Design review of the part built by this model. Coordinates are the model's own, in mm. A direction names the side the tool comes from. Coordinates: 2 decimals unless noted, no trailing zeros. Order: outer loops, then holes, each group sorted by start corner. A loop starts at its lowest first (then second) coordinate and runs counter-clockwise, first axis right, second up. Notation, with made-up numbers: (68, -26.75) - (108, -26.75) arc R8 ccw to (108, -13.75) - close; hole circle Ø2 at (-37, -38.5). An arc over 180 degrees is marked (long way). Write item = value, one per line. Start each with the question number.
```python
from build123d import *

# Parameters (mm, degrees)
SKETCH1_R               = 40
BOSS_EXTRUDE1_DEPTH     = 600
SHELL7_T                = 5
CUT_EXTRUDE2_DEPTH      = 40
CUT_EXTRUDE2_DEPTH_BACK = 40
SKETCH2_R               = 10


with BuildPart() as part:
    # Sketch1 → Boss-Extrude1 (new body)
    with BuildSketch(Plane(origin=(0, 0, 0), x_dir=(1, 0, 0), z_dir=(0, 1, 0))):
        with Locations(Location((0, 0, 0), (0, 0, 270))):
            Circle(SKETCH1_R)
    extrude(amount=BOSS_EXTRUDE1_DEPTH)

    # Shell7 (no face opened: a closed hollow body)
    add(offset(amount=-SHELL7_T, mode=Mode.PRIVATE), mode=Mode.SUBTRACT)

    # Sketch2 → Cut-Extrude2 (cut, two sides: drawn at the far end of the back side and taken through both)
    with BuildSketch(Plane.XY.offset(-CUT_EXTRUDE2_DEPTH_BACK)):
        with Locations(Location((0, 570, 0), (0, 0, 270))):
            Circle(SKETCH2_R)
    extrude(amount=CUT_EXTRUDE2_DEPTH + CUT_EXTRUDE2_DEPTH_BACK, mode=Mode.SUBTRACT)


solid = part.part
```
Item 1: Add section A-A on x = 0. Give the boundary of the cut face in (y, z), plus the area to 3 significant figures.
Item 2: For line 1 (Z direction, x = -1, y = 118.5); line 2 (X direction, y = 179, z = 0); line 3 (Y direction, x = 7, z = -7.5), list the stretches that pass through material, from the lowest coordinate up.
Item 3: For P1, Ø16, axis at x = 0, y = 570, coming from the -Z side; P2, Ø3, axis at x = 12.5, y = 272, coming from the -Z side; P3, Ø12, axis at y = 393, z = 20, coming from the +X side; P4, Ø5, axis at x = -26.5, y = 527.5, coming from the +Z side, all flat-tipped, find the tip position at first contact; note any pin that passes through.
Item 4: Add section B-B on z = 0. Give the boundary of the cut face in (x, y), plus the area to 3 significant figures.
Item 5: Add section D-D on y = 496. Give the boundary of the cut face in (x, z).
Item 6: Mouldability with a two-part tool opening along Y and no side actions: class faces 1 (the flat face through (1, 0, -1)), 2 (the flat face through (0, 5, 0)), 3 (the flat face through (1, 600, -1)) as +Y half, -Y half, draft (parallel to the pull), parting line (faces both ways), or undercut.
Item 7: For faces 4 (the cylindrical face through (-21, 296, -28)), 5 (the cylindrical face through (-8.872, 565.386, -36.816)), list the 3-axis set-ups (+Z, -Z, +X, -X, +Y, -Y) from which the entire face can be reached by the end or side of a thin tool; tool diameter is ignored.
Item 8: Add section C-C on x = -23. Give the boundary of the cut face in (y, z).
Worked out:
q1.outline = (0, -40) - (560, -40) - (560, -35) - (5, -35) - (5, 35) - (560, 35) - (560, 40) - (0, 40) - close; (580, -40) - (600, -40) - (600, 40) - (580, 40) - (580, 35) - (595, 35) - (595, -35) - (580, -35) - close
q1.area = 6,500 mm2
q2.line_1 = -39.99 to -34.99, 34.99 to 39.99
q2.line_2 = -40 to -35, 35 to 40
q2.line_3 = 0 to 5, 595 to 600
q3.P1 = through
q3.P2 = -38.46
q3.P3 = 37.47
q3.P4 = 32
q4.outline = (-40, 0) - (40, 0) - (40, 600) - (-40, 600) - close; hole (-35, 5) - (35, 5) - (35, 595) - (-35, 595) - close
q4.area = 6,700 mm2
q5.outline = circle Ø80 at (0, 0); hole circle Ø70 at (0, 0)
q6.face_1 = -Y half
q6.face_2 = undercut
q6.face_3 = +Y half
q7.face_4 = none
q7.face_5 = +Z, -Z
q8.outline = (0, -32.73) - (600, -32.73) - (600, 32.73) - (0, 32.73) - close; hole (5, -26.38) - (595, -26.38) - (595, 26.38) - (5, 26.38) - close
